Autodesk Inventor part; units mm, degrees
ref_plane "Plano de trabajo2" through (-10.2243, 33.4626, 0) normal (-1, 0, 0) x (0, 0, -1)
ref_plane "YZ Plane" through (0, 0, 0) normal (1, 0, 0) x (0, 1, 0)
ref_plane "XZ Plane" through (0, 0, 0) normal (0, 1, 0) x (-1, 0, 0)
sketch "Boceto3" plane through (0, 0, 0) normal (0, 0, 1) x (1, 0, 0)
  line L0 (-15.1624, 32.0626) -> (-18.8843, 32.0626)
  line L1 (-13.7243, 33.4626) -> (-13.7243, 30.9626)
  line L2 (-13.7243, 30.9626) -> (-14.4343, 30.9626)
  line L3 (-14.4343, 30.9626) -> (-15.1624, 32.0626)
  arc A0 (-18.8843, 32.0626) -> (-21.6243, 29.3226) centre (-18.8843, 29.3226) ccw
  line L4 (-13.7243, 33.4626) -> (-10.2243, 33.4626)
  line L5 (-21.6243, 29.3226) -> (-21.6243, 26.5626)
  arc A1 (-10.2243, 33.4626) -> (-10.2243, 26.5626) centre (5.1794, 30.0126) ccw
  line L6 (-21.6243, 26.5626) -> (-21.1243, 26.5626)
  line L7 (-10.2243, 26.5626) -> (-10.7243, 26.5626)
  arc A2 (-10.7243, 26.5626) -> (-21.1243, 26.5626) centre (-15.9243, 23.1493) ccw
  dimension "d218" = 2.5
  dimension "d219" = 0.71
  dimension "d221" = 33.5
  dimension "d223" = 2.74
  dimension "d281" = 3.5
  dimension "d288" = 2.76
  dimension "d291" = 0.5
  dimension "d292" = 0.5
extrude "Extrusión4" add sketch "Boceto3" against normal blind 587.4
ref_plane "Plano de trabajo2" through (-10.2243, 33.4626, 0) normal (-1, 0, 0) x (0, 0, -1)
ref_plane "Plano de trabajo4" through (0, 0, -293.7) normal (0, 0, 1) x (1, 0, 0)
sketch "Boceto5" plane through (-10.2243, 33.4626, 0) normal (-1, 0, 0) x (0, 0, -1)
  line L0 (0, 0) -> (0, 6.9)
  line L1 (0, 6.9) -> (6.9, 0)
  line L2 (0, 0) -> (587.4, 0)
  line L3 (6.9, 0) -> (0, 0)
  line L4 (0, 0) -> (0, 6.9)
  point P0 (0, 33.4626)
  dimension "d296" = 45
extrude "Extrusión6" cut sketch "Boceto5" along normal through all
mirror "Simetría3" about plane through (0, 0, -293.7) normal (0, 0, 1) of "Extrusión6"
properties part number "SP40-10 JUNTA INT CRISTAL 587 mm" material "Caucho"
The listing builds one solid part. Answer for the finished solid, in the listing's coordinates (mm). Round coordinates to 2 decimals unless told otherwise and drop trailing zeros. Loops run counter-clockwise (first coordinate to the right, second up) from the corner with the lowest first, then second, coordinate; pieces in that order, holes last.
Q1. Given pin 1 Ø1.3 at (y, z) = (33, -391.5) entering from -X; pin 2 Ø3 at (x, z) = (-18, -276.5) entering from +Y; pin 3 Ø1.5 at (x, z) = (-19.5, -104.5) entering from -Y; pin 4 Ø2 at (y, z) = (32.5, -380) entering from +X, each flat-ended and moving along its own axis, determine where each tip first touches the part or whether it passes through.
Q2. Section A-A, the plane y = 28 is taken. Determine the outline of the cut face in (x, z).
Q3. Find the intervals of material crossed by line 1 (X direction, y = 29.75, z = -37); line 2 (X direction, y = 31.25, z = -44); line 3 (Y direction, x = -10.75, z = -222.5), in increasing order.
Q4. Section B-B, the plane z = -181 is taken. Determine the outline of the cut face in (x, y), then the cut area to 3 significant figures.
Completed:
1. pin 1: stops at x = -13.72
1. pin 2: stops at y = 32.06
1. pin 3: stops at y = 27.62
1. pin 4: stops at x = -10.22
2. outline: (-21.62, -585.96) - (-19.82, -585.96) - (-19.82, -1.44) - (-21.62, -1.44) - close; (-12.03, -585.96) - (-10.48, -585.96) - (-10.48, -1.44) - (-12.03, -1.44) - close
3. line 1: x = -21.59 to -10.6
3. line 2: x = -20.83 to -14.62, -13.72 to -10.56
3. line 3: y = 26.6 to 33.46
4. outline: (-21.62, 26.56) - (-21.12, 26.56) arc R6.22 cw to (-10.72, 26.56) - (-10.22, 26.56) arc R15.79 cw to (-10.22, 33.46) - (-13.72, 33.46) - (-13.72, 30.96) - (-14.43, 30.96) - (-15.16, 32.06) - (-18.88, 32.06) arc R2.74 ccw to (-21.62, 29.32) - close
4. area: 42.5 mm2
